Work out the finished part from the listing and answer in its coordinate system (mm). Face numbers are marked on the shaded views. A direction names the side the tool comes from. Coordinates: 2 decimals unless noted, no trailing zeros. Order: outer loops, then holes, each group sorted by start corner. A loop starts at its lowest first (then second) coordinate and runs counter-clockwise, first axis right, second up. Notation, with made-up numbers: M 53,20.25 L 84,20.25 A15 cw 84,39.25 Z; hole C 0,-12.75 d11. An arc over 180 degrees is marked long. Answer in a Markdown table with one row per item. Add a question column.
Item 1: The part is cut by section A-A (z = 2.25). Write down the section's boundary in (x, y), then the cut area to 3 significant figures.
Item 2: Which of the six approach directions +Z, -Z, +X, -X, +Y, -Y give full straight-line access (tool end or side, diameter ignored) to the marked faces 4, 5 and 6?
Item 3: Flat-ended cylindrical pins translate along their axes: pin 1 Ø1.6 at (y, z) = (-7.5, 2.5) entering from +X; pin 2 Ø2 at (x, y) = (60.5, 8.5) entering from -Z; pin 3 Ø1 at (y, z) = (-7.5, 6.5) entering from -X. Find the tip coordinate at first contact, or state that the pin passes through.
Item 4: The part is cut by section D-D (x = 58.5). Write down the section's boundary in (y, z).
Item 5: Consider line 1 (Z direction, x = 60.75, y = -7.5); line 2 (X direction, y = -5, z = 1); line 3 (X direction, y = -8, z = 6.5). Determine where each line is inside the solid, lowest interval first. Write a range as from..to.
Item 6: The part is cut by section C-C (x = 60). Write down the section's boundary in (y, z).
Item 7: The part is cut by section B-B (y = -8.25). Write down the section's boundary in (x, z), then the cut area to 3 significant figures.
Item 8: The mould has two halves that part along Z. Classify the marked faces 1, 2 and 3: released by +Z, released by -Z, zero draft, split by the parting line, or undercut.
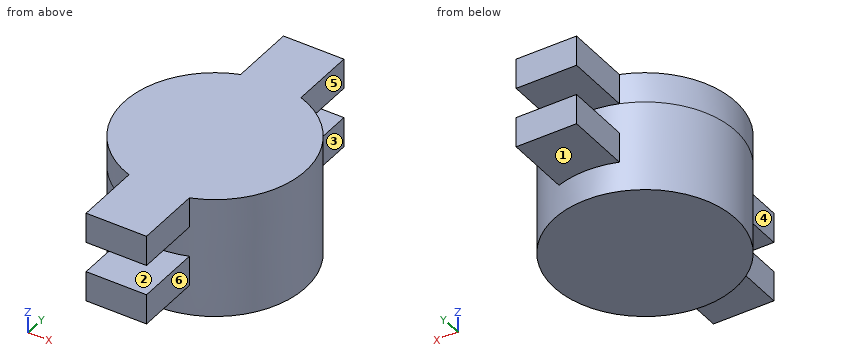
from build123d import *

# Parameters (mm, degrees)
SKETCH006_R      = 6
EXTRUDE006_DEPTH = 6
EXTRUDE007_DEPTH = 2
ARRAY001_Z_COUNT = 2
ARRAY001_Z_PITCH = 4


with BuildPart() as eixo2:
    # Sketch006 → Extrude006 (new body)
    with BuildSketch(Plane.XY):
        with Locations((60, 0)):
            Circle(SKETCH006_R)
    extrude(amount=EXTRUDE006_DEPTH)


with BuildPart() as obj1:
    # Sketch007 (on Face8 of Extrude002) → Extrude007 (new body)
    with BuildSketch(Plane.XY.offset(2)):
        with BuildLine():
            ThreePointArc((62, -5.6568542495), (66, 0), (62, 5.6568542495))
            Line((62, 5.6568542495), (62, 10))
            Line((58, 10), (62, 10))
            Line((58, 5.6568542495), (58, 10))
            ThreePointArc((58, 5.6568542495), (54, 0), (58, -5.6568542495))
            Line((58, -10), (58, -5.6568542495))
            Line((58, -10), (62, -10))
            Line((62, -5.6568542495), (62, -10))
        make_face()
    extrude(amount=EXTRUDE007_DEPTH)

    # Array001 Z: obj1 ×2


with BuildPart() as obj1_1:
    add(obj1.part)
    with Locations(*[(0, 0, i * ARRAY001_Z_PITCH) for i in range(1, ARRAY001_Z_COUNT)]):
        add(obj1.part)

    # Fusion: union Eixo2
    add(eixo2.part)


solid = obj1_1.part
Reply:
| question | item | result |
|---|---|---|
| 1 | outline | M 58,-10 L 62,-10 L 62,-5.66 A6 ccw 62,5.66 L 62,10 L 58,10 L 58,5.66 A6 ccw 58,-5.66 Z |
| 1 | area | 146 mm2 |
| 2 | face 4 | +Z, -Z, -X, -Y |
| 2 | face 5 | +Z, -Z, +X, +Y |
| 2 | face 6 | +Z, -Z, +X, -Y |
| 3 | pin 1 | stops at x = 62 |
| 3 | pin 2 | stops at z = 2 |
| 3 | pin 3 | stops at x = 58 |
| 4 | outline | M -10,2 L -5.81,2 L -5.81,0 L 5.81,0 L 5.81,2 L 10,2 L 10,4 L 5.81,4 L 5.81,6 L 10,6 L 10,8 L -10,8 L -10,6 L -5.81,6 L -5.81,4 L -10,4 Z |
| 5 | line 1 | z = 2..4, 6..8 |
| 5 | line 2 | x = 56.68..63.32 |
| 5 | line 3 | x = 58..62 |
| 6 | outline | M -10,2 L -6,2 L -6,0 L 6,0 L 6,2 L 10,2 L 10,4 L 6,4 L 6,6 L 10,6 L 10,8 L -10,8 L -10,6 L -6,6 L -6,4 L -10,4 Z |
| 7 | outline | M 58,2 L 62,2 L 62,4 L 58,4 Z; M 58,6 L 62,6 L 62,8 L 58,8 Z |
| 7 | area | 16.0 mm2 |
| 8 | face 1 | released by -Z |
| 8 | face 2 | undercut |
| 8 | face 3 | zero draft |
